Part print with two shaded views. Sizes in mm from the minimum x, y, z corner. Round coordinates to 2 decimals unless told otherwise and drop trailing zeros. Order: outer loops, then holes, each group sorted by start corner. A loop starts at its lowest first (then second) coordinate and runs counter-clockwise, first axis right, second up. Notation, with made-up numbers: (-6, 25.5) - (6, 25.5) arc R26 ccw to (6, 40.5) - close; hole circle Ø7 at (62, -32.75). An arc over 180 degrees is marked (long way). Answer as CSV lines item,"result". Start each with the question number.
1. Band-saw the part on C-C on y = 19.5. List the corners of the cut face in (x, z).
2. Band-saw the part on D-D on z = 1.5. List the corners of the cut face in (x, y).
3. Band-saw the part on B-B on x = 5.55. List the corners of the cut face in (y, z).
4. Wall check: line 1 along X through (y, z) = (36.55, 1.5); line 2 along Y through (x, z) = (36.5, 0.5); line 3 along X through (y, z) = (36, 5). Give the ranges that are in metal, low to high. Write a range as [from, to].
5. Band-saw the part on A-A on y = 36.55. List the corners of the cut face in (x, z).
6. Pin check, flat tip, straight feed: pin 1 Ø7 at (x, y) = (23, 15.5) entering from -Z. Stop position of the tip, or through.
7. Pull direction Y, two halves, no side cores. Call the marked faces 1, 2, 3 and 4: released by +Y, released by -Y, zero draft, split by the parting line, or undercut.
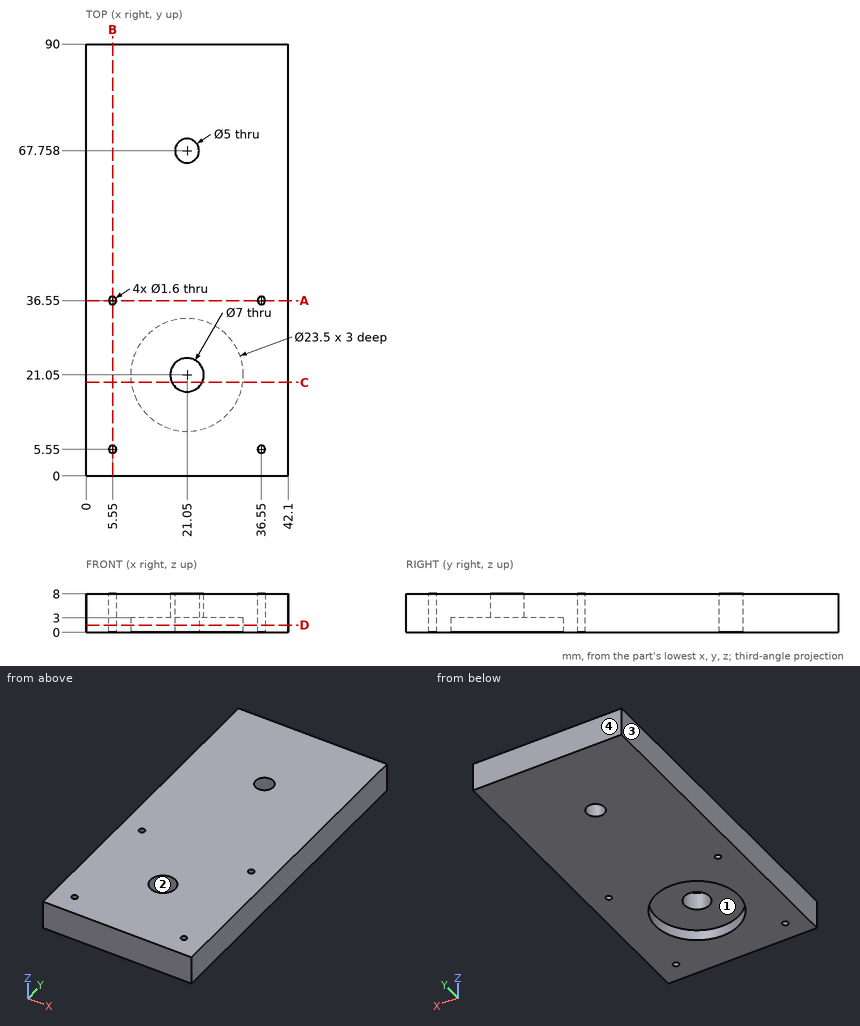
Reply:
1,outline,"(0, 0) - (9.4, 0) - (9.4, 3) - (17.91, 3) - (17.91, 8) - (0, 8) - close; (24.19, 3) - (32.7, 3) - (32.7, 0) - (42.1, 0) - (42.1, 8) - (24.19, 8) - close"
2,outline,"(0, 0) - (42.1, 0) - (42.1, 90) - (0, 90) - close; hole circle Ø1.6 at (5.55, 5.55); hole circle Ø1.6 at (5.55, 36.55); hole circle Ø23.5 at (21.05, 21.05); hole circle Ø5 at (21.05, 67.76); hole circle Ø1.6 at (36.55, 5.55); hole circle Ø1.6 at (36.55, 36.55)"
3,outline,"(0, 0) - (4.75, 0) - (4.75, 8) - (0, 8) - close; (6.35, 0) - (35.75, 0) - (35.75, 8) - (6.35, 8) - close; (37.35, 0) - (90, 0) - (90, 8) - (37.35, 8) - close"
4,line 1,"x = [0, 4.75], [6.35, 35.75], [37.35, 42.1]"
4,line 2,"y = [0, 4.75], [6.35, 35.75], [37.35, 90]"
4,line 3,"x = [0, 4.97], [6.13, 35.97], [37.13, 42.1]"
5,outline,"(0, 0) - (4.75, 0) - (4.75, 8) - (0, 8) - close; (6.35, 0) - (35.75, 0) - (35.75, 8) - (6.35, 8) - close; (37.35, 0) - (42.1, 0) - (42.1, 8) - (37.35, 8) - close"
6,pin 1,"stops at z = 3"
7,face 1,"undercut"
7,face 2,"undercut"
7,face 3,"zero draft"
7,face 4,"released by +Y"
